```python
from build123d import *

# Parameters (mm, degrees)
BOSS_EXTRUDE1_DEPTH = 1.5875
SKETCH2_W           = 37.592
SKETCH2_H           = 19.05
BOSS_EXTRUDE2_DEPTH = 0.635


with BuildPart() as part:
    # Sketch1 → Boss-Extrude1 (new, symmetric)
    with BuildSketch(Plane(origin=(0, 0, 0), x_dir=(1, 0, 0), z_dir=(0, 1, 0))):
        Polygon((-25.146, 0), (-18.796, 0), (-18.796, 19.05), (18.796, 19.05), (18.796, 0), (25.146, 0), (25.146, 25.4), (-25.146, 25.4), align=None)
    extrude(amount=BOSS_EXTRUDE1_DEPTH, both=True)

    # Sketch2 → Boss-Extrude2 (add, symmetric)
    with BuildSketch(Plane(origin=(0, 0, 0), x_dir=(1, 0, 0), z_dir=(0, 1, 0))):
        with Locations((0, 9.525)):
            Rectangle(SKETCH2_W, SKETCH2_H)
    extrude(amount=BOSS_EXTRUDE2_DEPTH, both=True)


solid = part.part
```
Geometry check sheet. Reference: the model listing, model coordinates, mm. A direction names the side the tool comes from. Round coordinates to 2 decimals unless told otherwise and drop trailing zeros. Order: outer loops, then holes, each group sorted by start corner. A loop starts at its lowest first (then second) coordinate and runs counter-clockwise, first axis right, second up. Notation, with made-up numbers: (88, -2) - (144, -2) arc R19 cw to (144, 14) - close; hole circle Ø2 at (30.25, -19). An arc over 180 degrees is marked (long way). Use a Markdown table: item, result. Add a question column.
(1) Depth check by flat-ended pin: pin 1 (5.5 mm diameter, centred on x = -6, z = -10, fed in from +Y) (3 decimals); pin 2 (1 mm diameter, centred on x = 4, z = -17.5, fed in from -Y) (3 decimals); pin 3 (0.5 mm diameter, centred on x = 2.5, y = 1, fed in from +Z). Enter the tip coordinate at first touch or a pass-through.
(2) Tool access check on faces 5 (the flat face through (0, 0, -25.4)), 6 (the flat face through (0, 0.635, -10)), 7 (the flat face through (-18.796, -1, -9)). Record the directions out of +Z, -Z, +X, -X, +Y, -Y that give a thin tool (end or side, any length) a straight path to the whole face; none if there is none.
(3) Release check for a two-part mould opening along X. For faces 1 (the flat face through (0, 1, -19.05)), 2 (the flat face through (0, -1, -19.05)), 3 (the flat face through (0, -1.588, -21)), 4 (the flat face through (-25.146, 0, -13)) record: pulls with the +X half, pulls with the -X half, needs draft (parallel to the pull), parting line crosses it, or undercut.
(4) Sectioned sample at A-A, the plane z = -6.75. Enter the section's corners in (x, y) (1 decimal).
(5) Material ranges on line 1 along X through (y, z) = (0.8, -12.25); line 2 along Y through (x, z) = (-14.5, -16) (3 decimals); line 3 along Z through (x, y) = (18.5, -1.3), recorded low to high. Write a range as [from, to].
Answers below:
| question | item | result |
|---|---|---|
| 1 | pin 1 | y = 0.635 |
| 1 | pin 2 | y = -0.635 |
| 1 | pin 3 | z = -19.05 |
| 2 | face 5 | -Z, +X, -X, +Y, -Y |
| 2 | face 6 | +Z, +Y |
| 2 | face 7 | +Z, -Y |
| 3 | face 1 | undercut |
| 3 | face 2 | undercut |
| 3 | face 3 | needs draft |
| 3 | face 4 | pulls with the -X half |
| 4 | outline | (-25.1, -1.6) - (-18.8, -1.6) - (-18.8, -0.6) - (18.8, -0.6) - (18.8, -1.6) - (25.1, -1.6) - (25.1, 1.6) - (18.8, 1.6) - (18.8, 0.6) - (-18.8, 0.6) - (-18.8, 1.6) - (-25.1, 1.6) - close |
| 5 | line 1 | [-25.15, -18.8], [18.8, 25.15] |
| 5 | line 2 | [-0.635, 0.635] |
| 5 | line 3 | [-25.4, -19.05] |
